from build123d import *

# Parameters (mm, degrees)
BOSS_EXTRUDE1_DEPTH      = 7.5
BOSS_EXTRUDE1_DEPTH_BACK = 7.5
FILLET1_R                = 10
FILLET2_R                = 10
CUT_EXTRUDE1_DEPTH       = 24.5


with BuildPart() as part:
    # Sketch1 → Boss-Extrude1 (new, two sides: drawn at the far end of the back side and taken through both)
    with BuildSketch(Plane(origin=(0, 0, 0), x_dir=(0, 0, -1), z_dir=(1, 0, 0)).offset(-BOSS_EXTRUDE1_DEPTH_BACK)):
        Polygon((0, 45), (0, 0), (5, 0), (5, 15), (10, 15), (10, 30), (15, 30), (15, 45), align=None)
    extrude(amount=BOSS_EXTRUDE1_DEPTH + BOSS_EXTRUDE1_DEPTH_BACK)

    # Fillet1
    # the kernel refuses this fillet: 10 mm, written as the material it takes off along each edge
    with BuildSketch(Plane(origin=(29.150635095, 30, -15), x_dir=(0, 1, 0), z_dir=(-1, 0, 0))) as fillet1_piece_1:
        with BuildLine():
            CenterArc((8.660254038, -10), FILLET1_R, 90, 60)
            Line((0, -5), (-0.173205081, -4.9))
            ThreePointArc((-0.173205081, -4.9), (-0.2, -2.5), (-0.2, 0))
            Line((-0.2, 0), (0, 0.2))
            Line((0, 0.2), (8.660254038, 0.2))
            Line((8.660254038, 0.2), (8.660254038, 0))
        make_face()
    extrude(amount=58.301270189, mode=Mode.SUBTRACT)

    # Fillet2
    # the kernel refuses this fillet: 10 mm, written as the material it takes off along each edge
    with BuildSketch(Plane(origin=(-29.150635095, 0, -5), x_dir=(0, 0, 1), z_dir=(1, 0, 0))) as fillet2_piece_1:
        with BuildLine():
            CenterArc((10, -8.660254038), FILLET2_R, 120, 60)
            Line((0, -8.660254038), (-0.2, -8.660254038))
            Line((-0.2, -8.660254038), (-0.2, 0))
            Line((-0.2, 0), (0, 0.2))
            ThreePointArc((0, 0.2), (2.5, 0.2), (4.9, 0.173205081))
            Line((4.9, 0.173205081), (5, 0))
        make_face()
    extrude(amount=58.301270189, mode=Mode.SUBTRACT)
    with BuildSketch(Plane(origin=(-29.150635095, 15, -10), x_dir=(0, 1, 0), z_dir=(1, 0, 0))) as fillet2_piece_2:
        with BuildLine():
            CenterArc((8.660254038, 10), FILLET2_R, 210, 60)
            Line((0, 5), (-0.173205081, 4.9))
            ThreePointArc((-0.173205081, 4.9), (-0.2, 2.5), (-0.2, 0))
            Line((-0.2, 0), (0, -0.2))
            Line((0, -0.2), (8.660254038, -0.2))
            Line((8.660254038, -0.2), (8.660254038, 0))
        make_face()
    extrude(amount=58.301270189, mode=Mode.SUBTRACT)

    # Sketch2 → Cut-Extrude1 (cut)
    with BuildSketch(Plane(origin=(7.5, 0, 0), x_dir=(0, 0, -1), z_dir=(1, 0, 0))):
        Polygon((-3.394371736, 45), (20.0100121, 45), (-5.085276302, 40.575023566), align=None)
    extrude(amount=-CUT_EXTRUDE1_DEPTH, mode=Mode.SUBTRACT)


solid = part.part
Check sheet for the modelled part. Datum: model origin and axes. Units: mm. A direction names the side the tool comes from. Give positions to 0.01 mm unless a question says otherwise; leave off trailing zeros. Write each loop counter-clockwise with the first axis right and the second up, starting at its lowest first coordinate (ties: lowest second). Pieces come first, ordered by that corner, then holes. Notation, with made-up numbers: (-30.5, 78.25) -> (-9.5, 78.25) arc R20 cw to (-9.5, 105.25) -> close; hole circle Ø3 at (-18, -33). An arc over 180 degrees is marked (long way). Write item = value, one per line.
Item 1: Scan lines: probe 1 along Z at (x, y) = (-6, 24.5); probe 2 along Z at (x, y) = (-6.25, 11.5); probe 3 along Y at (x, z) = (-2.75, -8). Record each from-to range of solid material in increasing order. Write a range as from..to.
Output:
probe_1 = -10..0
probe_2 = -5..0
probe_3 = 17.66..42.88
Item 2: Gauge pin test, flat ends, axial feed: pin 1 (5 mm diameter, centred on x = 0, y = 13.5, fed in from -Z); pin 2 (8 mm diameter, centred on x = 4.5, z = -12, fed in from -Y); pin 3 (7 mm diameter, centred on x = 3.5, y = 26, fed in from -Z). Record the tip position at first contact, or that the pin passes through.
Output:
pin_1 = -6.43
pin_2 = 17.66
pin_3 = -10
Item 3: Tool access check on faces 1 (the flat face through (0, 12, -5)), 2 (the flat face through (0, 21, 0)). Record the directions out of +Z, -Z, +X, -X, +Y, -Y that give a thin tool (end or side, any length) a straight path to the whole face; none if there is none.
Output:
face_1 = -Z, +X, -X, -Y
face_2 = +Z, +X, -X, +Y, -Y
Item 4: Sectioned sample at C-C on z = -8.5. Record the boundary of the cut face in (x, y).
Output:
outline = (-7.5, 18.39) -> (7.5, 18.39) -> (7.5, 42.97) -> (-7.5, 42.97) -> close
Item 5: Sectioned sample at B-B on y = 12. Record the boundary of the cut face in (x, z), and give its area (3 significant figures).
Output:
outline = (-7.5, -5) -> (7.5, -5) -> (7.5, 0) -> (-7.5, 0) -> close
area = 75.0 mm^2
Item 6: Sectioned sample at A-A on x = 4.25. Record the boundary of the cut face in (y, z).
Output:
outline = (0, 0) arc R10 ccw to (8.66, -5) -> (15, -5) arc R10 ccw to (23.66, -10) -> (30, -10) arc R10 ccw to (38.66, -15) -> (44.12, -15) -> (41.47, 0) -> close
